```python
from build123d import *

# Parameters (mm, degrees)
ESBO_O1_W                  = 22
ESBO_O1_H                  = 22
RESSALTO_EXTRUS_O1_DEPTH   = 24.25
RESSALTO_EXTRUS_O1_2_DEPTH = 24.25
ESBO_O2_R                  = 11
RESSALTO_EXTRUS_O2_DEPTH   = 15
CORTE_EXTRUS_O1_DEPTH      = 65.730692102
CORTE_EXTRUS_O1_DEPTH_BACK = 65.730692102
ESBO_O4_R                  = 0.75
RESSALTO_EXTRUS_O3_DEPTH   = 3


with BuildPart() as part:
    # Esbo_o1 → Ressalto-extrus_o1 (new, symmetric)
    with BuildSketch(Plane.XY):
        Rectangle(ESBO_O1_W, ESBO_O1_H)
    extrude(amount=RESSALTO_EXTRUS_O1_DEPTH, both=True)



with BuildPart() as body_2:
    # Esbo_o1 → Ressalto-extrus_o1 2 (new, symmetric)
    with BuildSketch(Plane.XY):
        with Locations((37, 0)):
            Rectangle(ESBO_O1_W, ESBO_O1_H)
    extrude(amount=RESSALTO_EXTRUS_O1_2_DEPTH, both=True)


with BuildPart() as part_1:
    add(part.part)

    add(body_2.part)  # Ressalto-extrus_o2 merges body 2
    # Esbo_o2 → Ressalto-extrus_o2 (add)
    with BuildSketch(Plane(origin=(11, 0, 0), x_dir=(0, 0, -1), z_dir=(1, 0, 0))):
        with Locations(Location((0.75, 0, 0), (0, 0, 270))):
            Circle(ESBO_O2_R)
    extrude(amount=RESSALTO_EXTRUS_O2_DEPTH)

    # Esbo_o3 → Corte-extrus_o1 (cut, two sides)
    with BuildSketch(Plane(origin=(48, 0, 0), x_dir=(0, 0, -1), z_dir=(1, 0, 0))) as corte_extrus_o1_sk:
        with BuildLine():
            Line((0.75, 11), (24.25, 11))
            Line((24.25, 11), (24.25, -11))
            Line((24.25, -11), (0.75, -11))
            ThreePointArc((0.75, -11), (11.75, 0), (0.75, 11))
        make_face()
    extrude(amount=CORTE_EXTRUS_O1_DEPTH, mode=Mode.SUBTRACT)
    extrude(corte_extrus_o1_sk.sketch, amount=-CORTE_EXTRUS_O1_DEPTH_BACK, mode=Mode.SUBTRACT)

    # Esbo_o4 → Ressalto-extrus_o3 (add)
    with BuildSketch(Plane.XY.offset(24.25)):
        with Locations((-5.5, 0)):
            Circle(ESBO_O4_R)
        with Locations((2.5, 0)):
            Circle(ESBO_O4_R)
        with Locations((-1.5, 8)):
            Circle(ESBO_O4_R)
        with Locations((-1.5, -8)):
            Circle(ESBO_O4_R)
        with Locations((34.5, 0)):
            Circle(ESBO_O4_R)
        with Locations((42.5, 0)):
            Circle(ESBO_O4_R)
        with Locations((38.5, -8)):
            Circle(ESBO_O4_R)
        with Locations((38.5, 8)):
            Circle(ESBO_O4_R)
    extrude(amount=RESSALTO_EXTRUS_O3_DEPTH)


solid = part_1.part
```
Design review of the part built by this model. Coordinates are the model's own, in mm. A direction names the side the tool comes from. Coordinates: 2 decimals unless noted, no trailing zeros. Write each loop counter-clockwise with the first axis right and the second up, starting at its lowest first coordinate (ties: lowest second). Pieces come first, ordered by that corner, then holes.
1) To check wall thickness, follow L1, parallel to X at y = 8.5, z = 21; L2, parallel to Z at x = 28.5, y = 0; L3, parallel to X at y = 7.75, z = 24.5. State the ranges of each line that lie inside material, in increasing order.
2) Add section D-D (z = 4.5). Write out the cut boundary in (x, y).
3) Add section B-B (x = -5.5). Write out the cut boundary in (y, z).
4) Insertion check: pin 1 (6 mm diameter, centred on x = 8, y = 4.5, fed in from +Z); pin 2 (11 mm diameter, centred on x = -4, y = -0.5, fed in from +Z); pin 3 (2 mm diameter, centred on x = 22, y = 7.5, fed in from +Z). Each pin has a flat end and moves straight along its axis. Give the tip position at first contact, or say it passes through.
5) Add section C-C (y = 0). Write out the cut boundary in (x, z), plus the area to 3 significant figures.
6) Machinability: for faces 3 (the flat face through (34, 0, 27.25)), 4 (the cylindrical face through (18.087, 1.432, -11.656)), 5 (the cylindrical face through (-0.785, -7.775, 25.729)), which of the approach directions +Z, -Z, +X, -X, +Y, -Y give a long, thin tool a straight path to every point of the face, cutting with its end or side? Answer none if there is none.
7) Add section A-A (z = 13). Write out the cut boundary in (x, y), plus the area to 3 significant figures.
8) Mouldability with a two-part tool opening along X and no side actions: class faces 1 (the flat face through (-2, 8, 27.25)), 2 (the flat face through (26, 0, 17)) as +X half, -X half, draft (parallel to the pull), parting line (faces both ways), or undercut.
Check result:
1. L1: x = -11 to 11, 26 to 48
1. L2: z = -11.75 to 24.25
1. L3: x = -2.21 to -0.79, 37.79 to 39.21
2. outline: (-11, -11) - (11, -11) - (11, -9.67) - (26, -9.67) - (26, -11) - (48, -11) - (48, 11) - (26, 11) - (26, 9.67) - (11, 9.67) - (11, 11) - (-11, 11) - close
3. outline: (-11, -0.75) arc R11 ccw to (11, -0.75) - (11, 24.25) - (0.75, 24.25) - (0.75, 27.25) - (-0.75, 27.25) - (-0.75, 24.25) - (-11, 24.25) - close
4. pin 1: stops at z = 24.25
4. pin 2: stops at z = 27.25
4. pin 3: stops at z = 8.12
5. outline: (-11, -11.75) - (48, -11.75) - (48, 24.25) - (43.25, 24.25) - (43.25, 27.25) - (41.75, 27.25) - (41.75, 24.25) - (35.25, 24.25) - (35.25, 27.25) - (33.75, 27.25) - (33.75, 24.25) - (26, 24.25) - (26, 10.25) - (11, 10.25) - (11, 24.25) - (3.25, 24.25) - (3.25, 27.25) - (1.75, 27.25) - (1.75, 24.25) - (-4.75, 24.25) - (-4.75, 27.25) - (-6.25, 27.25) - (-6.25, 24.25) - (-11, 24.25) - close
5. area: 1,930 mm2
6. face 3: +Z, +X, -X, +Y, -Y
6. face 4: none
6. face 5: +Z
7. outline: (-11, -11) - (11, -11) - (11, 11) - (-11, 11) - close; (26, -11) - (48, -11) - (48, 11) - (26, 11) - close
7. area: 968 mm2
8. face 1: draft
8. face 2: undercut
